from build123d import *

# Parameters (mm, degrees)
BOSS_EXTRUDE1_DEPTH            = 2.286
F_3_16_0_1875_DIAMETER_HOLE1_D = 4.7625


with BuildPart() as part:
    # Sketch1 → Boss-Extrude1 (new body)
    with BuildSketch(Plane(origin=(0, 0, 0), x_dir=(1, 0, 0), z_dir=(0, 1, 0))):
        Polygon((-25.4, 76.30478401), (-25.4, 25.4), (0, 25.4), (0, 0), (-50.8, 0), (-50.8, 76.30478401), align=None)
    extrude(amount=BOSS_EXTRUDE1_DEPTH)

    # 3/16 (0.1875) Diameter Hole1 (through all)
    with Locations(Plane(origin=(0, 2.286, 0), x_dir=(1, 0, 0), z_dir=(0, 1, 0))):
        with Locations((-38.1, 63.60478401), (-38.1, 38.20478401), (-38.1, 12.7), (-12.7, 12.7)):
            Hole(F_3_16_0_1875_DIAMETER_HOLE1_D / 2)


solid = part.part
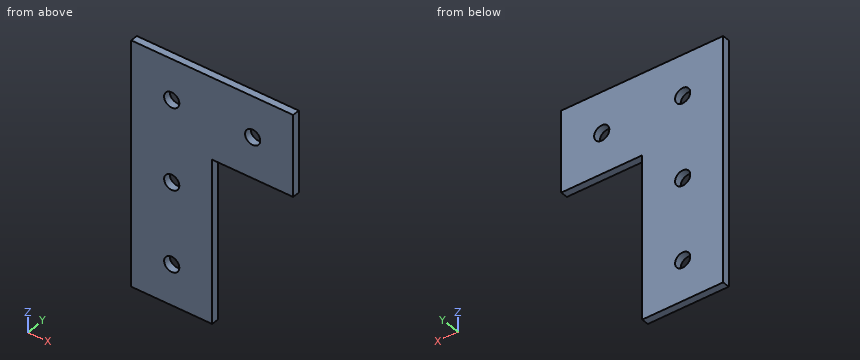
Design review of the part built by this model. Coordinates are the model's own, in mm. Give positions to 0.01 mm unless a question says otherwise; leave off trailing zeros. Loops run counter-clockwise (first coordinate to the right, second up) from the corner with the lowest first, then second, coordinate; pieces in that order, holes last. Notation, with made-up numbers: (-14.5, -2) - (26.5, -2) arc R10 ccw to (26.5, 6) - close; hole circle Ø8 at (10.25, 59). An arc over 180 degrees is marked (long way). Write item = value, one per line.
1) Take a section at C-C on x = -38.1. State the section outline as (y, z) points, and give its area (3 significant figures).
Result sheet:
outline = (0, -76.3) - (2.29, -76.3) - (2.29, -65.99) - (0, -65.99) - close; (0, -61.22) - (2.29, -61.22) - (2.29, -40.59) - (0, -40.59) - close; (0, -35.82) - (2.29, -35.82) - (2.29, -15.08) - (0, -15.08) - close; (0, -10.32) - (2.29, -10.32) - (2.29, 0) - (0, 0) - close
area = 142 mm2
2) Clearance check with flat-ended pins moving along their axes: pin 1 Ø5.5 at (x, z) = (-38.1, -38.2) entering from -Y; pin 2 Ø1.1 at (x, y) = (-8.5, 1) entering from -Z; pin 3 Ø0.7 at (y, z) = (0.5, -52.5) entering from +X. State where each tip first meets the part, or that it passes through.
Result sheet:
pin_1 = 0
pin_2 = -25.4
pin_3 = -25.4
3) Take a section at A-A on x = -12.7. State the section outline as (y, z) points.
Result sheet:
outline = (0, -25.4) - (2.29, -25.4) - (2.29, -15.08) - (0, -15.08) - close; (0, -10.32) - (2.29, -10.32) - (2.29, 0) - (0, 0) - close
4) Take a section at D-D on y = 1.3. State the section outline as (x, z) points.
Result sheet:
outline = (-50.8, -76.3) - (-25.4, -76.3) - (-25.4, -25.4) - (0, -25.4) - (0, 0) - (-50.8, 0) - close; hole circle Ø4.76 at (-38.1, -63.6); hole circle Ø4.76 at (-38.1, -38.2); hole circle Ø4.76 at (-38.1, -12.7); hole circle Ø4.76 at (-12.7, -12.7)
5) To check wall thickness, follow line 1 (Z direction, x = -38.1, y = 0.65); line 2 (Z direction, x = -12.7, y = 0.6); line 3 (X direction, y = 1.15, z = -12.7). State the ranges of each line that lie inside material, in increasing order.
Result sheet:
line_1 = -76.3 to -65.99, -61.22 to -40.59, -35.82 to -15.08, -10.32 to 0
line_2 = -25.4 to -15.08, -10.32 to 0
line_3 = -50.8 to -40.48, -35.72 to -15.08, -10.32 to 0
6) Take a section at B-B on z = -12.7. State the section outline as (x, y) points.
Result sheet:
outline = (-50.8, 0) - (-40.48, 0) - (-40.48, 2.29) - (-50.8, 2.29) - close; (-35.72, 0) - (-15.08, 0) - (-15.08, 2.29) - (-35.72, 2.29) - close; (-10.32, 0) - (0, 0) - (0, 2.29) - (-10.32, 2.29) - close
